from build123d import *

# Parameters (mm, degrees)
BOSS_EXTRUDE1_DEPTH        = 2.5
BOSS_EXTRUDE1_DEPTH_BACK   = 2.5
SKETCH1_R                  = 2
SKETCH1_R_2                = 1.25
BOSS_EXTRUDE1_2_DEPTH      = 2.5
BOSS_EXTRUDE1_2_DEPTH_BACK = 2.5


with BuildPart() as part:
    # Sketch1 → Boss-Extrude1 (new, two sides: drawn at the far end of the back side and taken through both)
    with BuildSketch(Plane.XY.offset(-BOSS_EXTRUDE1_DEPTH_BACK)):
        Circle(SKETCH1_R)
        Circle(SKETCH1_R_2, mode=Mode.SUBTRACT)
    extrude(amount=BOSS_EXTRUDE1_DEPTH + BOSS_EXTRUDE1_DEPTH_BACK)



with BuildPart() as body_2:
    # Sketch1 → Boss-Extrude1 2 (new, two sides: drawn at the far end of the back side and taken through both)
    with BuildSketch(Plane.XY.offset(-BOSS_EXTRUDE1_2_DEPTH_BACK)):
        with Locations((67.5, 0)):
            Circle(SKETCH1_R)
        with Locations((67.5, 0)):
            Circle(SKETCH1_R_2, mode=Mode.SUBTRACT)
    extrude(amount=BOSS_EXTRUDE1_2_DEPTH + BOSS_EXTRUDE1_2_DEPTH_BACK)


with BuildPart() as part_1:
    add(part.part)

    add(body_2.part)  # Revolve3 merges body 2
    # Sketch2 → Revolve3 (revolve)
    with BuildSketch(Plane.XY, mode=Mode.PRIVATE) as revolve3_sk:
        with BuildLine():
            ThreePointArc((65.5, 0), (65.568148347, 0.51763809), (65.767949192, 1))
            Line((65.767949192, 1), (1.732050808, 1))
            ThreePointArc((1.732050808, 1), (1.931851653, 0.51763809), (2, 0))
            Line((2, 0), (2.240774351, 0))
            Line((2.240774351, 0), (65.5, 0))
        make_face()
    revolve(revolve3_sk.sketch.rotate(Axis((2, 0, 0), (1, 0, 0)), 90), axis=Axis((2, 0, 0), (1, 0, 0)))


solid = part_1.part
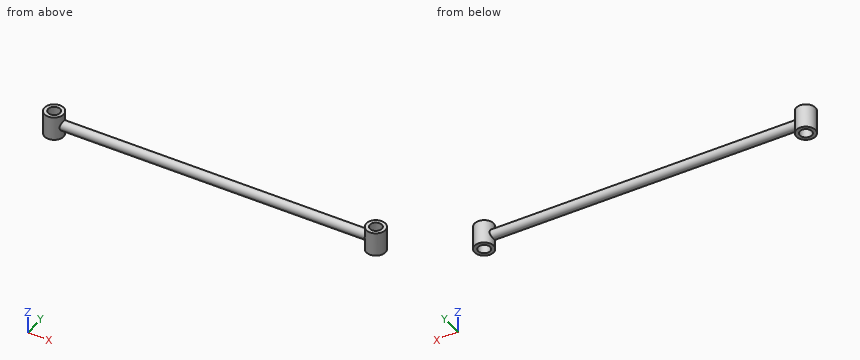
For this review, take the finished solid that the model builds, in its own axes (mm). Round coordinates to 2 decimals unless told otherwise and drop trailing zeros. Loops run counter-clockwise (first coordinate to the right, second up) from the corner with the lowest first, then second, coordinate; pieces in that order, holes last. Notation, with made-up numbers: (-11, -4.5) - (22, -4.5) arc R28 cw to (22, 17.5) - close; hole circle Ø9 at (50, 31.5). An arc over 180 degrees is marked (long way). Put each result on its own line as item: value. Start each with the question number.
1. Consider section A-A on x = 67.5. State the section outline as (y, z) points.
2. Consider section B-B on z = 1.75. State the section outline as (x, y) points.
3. For probe 1 along X at (y, z) = (-0.15, 1.7); probe 2 along X at (y, z) = (-0.05, -0.1); probe 3 along Y at (x, z) = (67.5, 0.6), list the stretches that pass through material, from the lowest coordinate up. Write a range as [from, to].
Result sheet:
1. outline: (-2, -2.5) - (-1.25, -2.5) - (-1.25, 2.5) - (-2, 2.5) - close; (1.25, -2.5) - (2, -2.5) - (2, 2.5) - (1.25, 2.5) - close
2. outline: circle Ø4 at (0, 0); circle Ø4 at (67.5, 0); hole circle Ø2.5 at (0, 0); hole circle Ø2.5 at (67.5, 0)
3. probe 1: [-1.99, -1.24], [1.24, 1.99], [65.51, 66.26], [68.74, 69.49]
3. probe 2: [-2, -1.25], [1.25, 66.25], [68.75, 69.5]
3. probe 3: [-2, -1.25], [1.25, 2]
